Design review of the part built by this model. Coordinates are the model's own, in mm. A direction names the side the tool comes from. Coordinates: 2 decimals unless noted, no trailing zeros. Write each loop counter-clockwise with the first axis right and the second up, starting at its lowest first coordinate (ties: lowest second). Pieces come first, ordered by that corner, then holes.
```python
from build123d import *

# Parameters (mm, degrees)
SKETCH4_R          = 99
CUT_EXTRUDE1_DEPTH = 1
CUT_EXTRUDE2_START = -74
CUT_EXTRUDE2_DEPTH = 74
CUT_EXTRUDE3_REACH = 161.612
CIRPATTERN1_COUNT  = 8


# Read off the part's stored shape, not the designer's step: Cut-Extrude2
with BuildPart() as part:
    # Sketch1 → Revolve1 (revolve)
    with BuildSketch(Plane.XY, mode=Mode.PRIVATE) as revolve1_sk:
        Polygon((0, 0), (-100, 0), (-100, -20), (-45, -51.754264805), (-45, -75), (-25, -75), (-25, -2), (0, -2), align=None)
    revolve(revolve1_sk.sketch.rotate(Axis((0, 0, 0), (0, 1, 0)), 270), axis=Axis((0, 0, 0), (0, 1, 0)))

    # Sketch4 → Cut-Extrude1 (cut)
    with BuildSketch(Plane(origin=(0, 0, 0), x_dir=(1, 0, 0), z_dir=(0, 1, 0))):
        with Locations(Location((0, 0, 0), (0, 0, 270))):
            Circle(SKETCH4_R)
    extrude(amount=-CUT_EXTRUDE1_DEPTH, mode=Mode.SUBTRACT)

    # Cut-Extrude2 outline → Cut-Extrude2 (cut)
    with BuildSketch(Plane(origin=(0, -1, 0), x_dir=(1, 0, 0), z_dir=(0, 1, 0)).offset(CUT_EXTRUDE2_START)):
        with BuildLine():
            ThreePointArc((-24.190856768, -9.529031895), (-26, 0), (-24.190856768, 9.529031895))
            Line((-24.190856768, 9.529031895), (-40.938372991, 16.126053976))
            ThreePointArc((-40.938372991, 16.126053976), (-44, 0), (-40.938372991, -16.126053976))
            Line((-40.938372991, -16.126053976), (-24.190856768, -9.529031895))
        make_face()
    cut_extrude2 = extrude(amount=CUT_EXTRUDE2_DEPTH, mode=Mode.SUBTRACT)

    # Cut-Extrude3: up to this cone (the profile starts inside it)
    cut_extrude3_end = Plane(origin=(0, -1, 0), z_dir=(0, 1, 0)).offset(-74.425624842) * Cone(1.732e-06, 632.972063387, 365.446590186, align=(Align.CENTER, Align.CENTER, Align.MIN), mode=Mode.PRIVATE)
    # Sketch5<4> → Cut-Extrude3 (cut, up to the surface)
    with BuildSketch(Plane(origin=(0, -1, 0), x_dir=(1, 0, 0), z_dir=(0, 1, 0)), mode=Mode.PRIVATE) as cut_extrude3_sk1:
        with BuildLine():
            Line((-88.389668958, -34.817616539), (-24.190856768, -9.529031895))
            ThreePointArc((-24.190856768, -9.529031895), (-26, 0), (-24.190856768, 9.529031895))
            Line((-24.190856768, 9.529031895), (-88.389668958, 34.817616539))
            ThreePointArc((-88.389668958, 34.817616539), (-95, 0), (-88.389668958, -34.817616539))
        make_face()
    cut_extrude3_tool1 = extrude(cut_extrude3_sk1.sketch, amount=-CUT_EXTRUDE3_REACH, mode=Mode.PRIVATE) & cut_extrude3_end
    cut_extrude3 = cut_extrude3_tool1.solids().sort_by_distance((-65.495165, -1, 0))[0]
    add(cut_extrude3, mode=Mode.SUBTRACT)

    # CirPattern1: Cut-Extrude2, Cut-Extrude3 ×8 about axis
    cirpattern1_axis = Axis((0, 0, 0), (0, 1, 0))
    add([cut_extrude2.rotate(cirpattern1_axis, i * 360 / CIRPATTERN1_COUNT) for i in range(1, CIRPATTERN1_COUNT)], mode=Mode.SUBTRACT)
    add([cut_extrude3.rotate(cirpattern1_axis, i * 360 / CIRPATTERN1_COUNT) for i in range(1, CIRPATTERN1_COUNT)], mode=Mode.SUBTRACT)


solid = part.part
```
(1) Consider section B-B (z = 0). Give the boundary of the cut face in (x, y), plus the area to 3 significant figures.
(2) Wall thickness on line 1 (X direction, y = -57.5, z = 38.5); line 2 (Z direction, x = 53.5, y = -7); line 3 (Z direction, x = -82, y = -8): over which ranges is each line inside the solid? List them lowest first.
(3) Consider section A-A (x = 0). Give the boundary of the cut face in (y, z), plus the area to 3 significant figures.
(4) Mouldability with a two-part tool opening along Z and no side actions: class faces 3 (the cylindrical face through (17.235, -63.54, -41.569)), 4 (the cylindrical face through (0, -63, -44)), 5 (the flat face through (-23, 0, -97)) as +Z half, -Z half, draft (parallel to the pull), parting line (faces both ways), or undercut.
(5) For faces 1 (the cylindrical face through (67.53, -10.65, -66.82)), 2 (the cylindrical face through (30.949, -62.686, 31.276)), list the 3-axis set-ups (+Z, -Z, +X, -X, +Y, -Y) from which the entire face can be reached by the end or side of a thin tool; tool diameter is ignored.
(6) Insertion check: pin 1 Ø10 at (y, z) = (-63, 40.5) entering from +X; pin 2 Ø1 at (y, z) = (-60.5, -20) entering from +X; pin 3 Ø8 at (x, z) = (72.5, 26.5) entering from +Y. Each pin has a flat end and moves straight along its axis. Give the tip position at first contact, or say it passes through.
(7) Consider section C-C (y = -67.5). State how many separate pieces and enclosed holes the cut face has, plus the area to 3 significant figures.
Results:
1. outline: (-100, -20) - (-45, -51.75) - (-45, -75) - (-44, -75) - (-44, -50.02) - (-95, -20.58) - (-95, -1) - (-99, -1) - (-99, 0) - (-100, 0) - close; (-26, -75) - (-25, -75) - (-25, -2) - (25, -2) - (25, -75) - (26, -75) - (26, -1) - (-26, -1) - close; (44, -75) - (45, -75) - (45, -51.75) - (100, -20) - (100, 0) - (99, 0) - (99, -1) - (95, -1) - (95, -20.58) - (44, -50.02) - close
1. area: 686 mm2
2. line 1: x = -23.3 to -21.3, -16.74 to -15.17, 15.17 to 16.74, 21.3 to 23.3
2. line 2: z = -84.49 to -78.5, -23.26 to -21.07, 21.07 to 23.26, 78.5 to 84.49
2. line 3: z = -57.24 to -47.97, -35.65 to -32.3, 32.3 to 35.65, 47.97 to 57.24
3. outline: (-75, -45) - (-51.75, -45) - (-20, -100) - (0, -100) - (0, -99) - (-1, -99) - (-1, -95) - (-20.58, -95) - (-50.02, -44) - (-75, -44) - close; (-75, -26) - (-1, -26) - (-1, 26) - (-75, 26) - (-75, 25) - (-2, 25) - (-2, -25) - (-75, -25) - close; (-75, 44) - (-50.02, 44) - (-20.58, 95) - (-1, 95) - (-1, 99) - (0, 99) - (0, 100) - (-20, 100) - (-51.75, 45) - (-75, 45) - close
3. area: 686 mm2
4. face 3: parting line
4. face 4: undercut
4. face 5: draft
5. face 1: +Y
5. face 2: +Y, -Y
6. pin 1: stops at x = 27.65
6. pin 2: stops at x = 40.56
6. pin 3: stops at y = -1
7. separate pieces: 1
7. enclosed holes: 9
7. area: 616 mm2
